Geometry: final body of the model. Coordinates: model frame, mm. Round coordinates to 2 decimals unless told otherwise and drop trailing zeros. Write each loop counter-clockwise with the first axis right and the second up, starting at its lowest first coordinate (ties: lowest second). Pieces come first, ordered by that corner, then holes. Notation, with made-up numbers: (-37, -7) - (-6, -7) arc R12 cw to (-6, 2) - close; hole circle Ø8 at (8, 19.25). An arc over 180 degrees is marked (long way). Use a Markdown table: item, result. Add a question column.
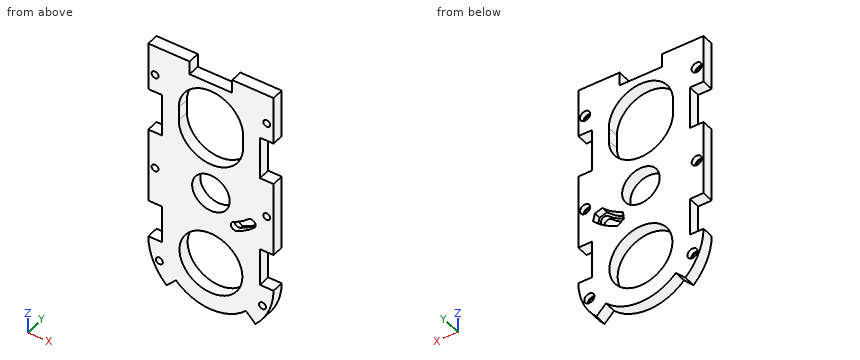
Autodesk Inventor part; units mm, degrees
ref_plane "YZ Plane" through (0, 0, 0) normal (1, 0, 0) x (0, 1, 0)
ref_plane "XZ Plane" through (0, 0, 0) normal (0, 1, 0) x (-1, 0, 0)
ref_plane "XY Plane" through (0, 0, 0) normal (0, 0, 1) x (1, 0, 0)
sketch "Boceto1" plane through (0, 0, 0) normal (0, 1, 0) x (-1, 0, 0)
  line L0 (0, 0) -> (-24.6, 0)
  line L1 (0, 0) -> (0, -29)
  line L2 (0, -29) -> (-8, -29)
  line L3 (-8, -29) -> (-8, -54)
  line L4 (-8, -54) -> (0, -54)
  line L5 (0, -54) -> (0, -99)
  line L6 (0, -99) -> (-8, -99)
  line L7 (-8, -99) -> (-8, -121)
  line L8 (-8, -121) -> (0, -121)
  line L9 (-24.6, 0) -> (-24.6, -8)
  line L10 (-24.6, -8) -> (-49.4, -8)
  line L11 (-37, 21.7087) -> (-37, -150)
  arc A0 (-57.5061, -141.5061) -> (-16.4939, -141.5061) centre (-37, -121) ccw
  line L12 (-37, -121) -> (-16.4939, -141.5061)
  line L13 (-16.4939, -141.5061) -> (-10.837, -147.163)
  line L14 (-74, 0) -> (-49.4, 0)
  line L15 (-74, 0) -> (-74, -29)
  line L16 (-74, -29) -> (-66, -29)
  line L17 (-66, -29) -> (-66, -54)
  line L18 (-66, -54) -> (-74, -54)
  line L19 (-74, -54) -> (-74, -99)
  line L20 (-74, -99) -> (-66, -99)
  line L21 (-66, -99) -> (-66, -121)
  line L22 (-66, -121) -> (-74, -121)
  line L23 (-49.4, 0) -> (-49.4, -8)
  line L24 (-37, -121) -> (-57.5061, -141.5061)
  line L25 (-57.5061, -141.5061) -> (-63.163, -147.163)
  arc A1 (-74, -121) -> (-63.163, -147.163) centre (-37, -121) ccw
  arc A2 (-10.837, -147.163) -> (0, -121) centre (-37, -121) ccw
  dimension "d139" = 24.6
  dimension "d140" = 29
  dimension "d141" = 25
  dimension "d142" = 8
  dimension "d143" = 45
  dimension "d144" = 22
  dimension "d145" = 8
  dimension "d146" = 24.8
  dimension "d148" = 45
extrude "Extrusión1" add sketch "Boceto1" along normal blind 7
sketch "Boceto2" plane through (0, 7, 0) normal (0, 1, 0) x (1, 0, 0)
  arc A0 (18, 32) -> (56, 32) centre (37, 32) ccw
  arc A1 (56, 40) -> (18, 40) centre (37, 40) ccw
  line L0 (18, 40) -> (18, 32)
  line L1 (56, 32) -> (56, 40)
  circle A2 centre (37, 77) radius 11.1
  circle A3 centre (37, 121) radius 18.6
  line L2 (37, -3.2334) -> (37, 158.5758)
  point P0 (0, 0)
  dimension "d18" = 19
  dimension "d23" = 22.2
  dimension "d25" = 37.2
  dimension "d149" = 44
  dimension "d150" = 37
  dimension "d151" = 8
extrude "Extrusión2" cut sketch "Boceto2" against normal blind 7
sketch "Boceto3" plane through (0, 7, 0) normal (0, 1, 0) x (1, 0, 0)
  line L0 (37, -12.6618) -> (37, 178.5268)
  circle A0 centre (4, 18) radius 2.05
  circle A1 centre (4, 76.5) radius 2.05
  circle A2 centre (37, 121) radius 18.6
  circle A3 centre (37, 121) radius 33
  circle A4 centre (6.512, 133.6286) radius 2.05
  line L1 (8, 29) -> (0, 29)
  line L2 (0, 29) -> (0, 0)
  line L3 (0, 99) -> (0, 54)
  line L4 (8, 99) -> (0, 99)
  line L5 (6.512, 133.6286) -> (37, 121)
  line L6 (24.8695, 121) -> (50.3921, 121)
  circle A5 centre (70, 18) radius 2.05
  circle A6 centre (70, 76.5) radius 2.05
  circle A7 centre (67.488, 133.6286) radius 2.05
  line L7 (67.488, 133.6286) -> (37, 121)
  dimension "d157" = 66
  dimension "d152" = 11
  dimension "d153" = 4
  dimension "d154" = 4.1
  dimension "d155" = 4
  dimension "d156" = 22.5
  dimension "d158" = 22.5
extrude "Extrusión3" cut sketch "Boceto3" against normal through all contours A4 A3 | A3 L5 A4 | A3 A4 L5 | A7 L7 A3 | A3 A7 | L7 A7 A3 | A0 | A1 | A5 | A6
sketch "Boceto12" plane through (0, 7, 0) normal (0, 1, 0) x (1, 0, 0)
  circle A0 centre (37, 77) radius 11.1
  circle A1 centre (37, 121) radius 18.6
  arc A2 (60.7956, 85.0881) -> (51.3765, 91.3074) centre (38.4503, 61.4886) ccw
  line L0 (38.4503, 61.4886) -> (60.7956, 85.0881)
  line L1 (38.4503, 61.4886) -> (51.3765, 91.3074)
  line L2 (51.3765, 91.3074) -> (52.4106, 93.693)
  line L3 (60.7956, 85.0881) -> (62.5832, 86.9761)
  line L4 (38.4503, 61.4886) -> (51.3765, 91.3074)
  line L5 (50.3411, 88.9225) -> (50.3424, 88.9219)
  line L6 (59.009, 83.1992) -> (59.008, 83.2002)
  circle A3 centre (51.3765, 91.3074) radius 2.6
  circle A4 centre (60.7956, 85.0881) radius 2.6
  circle A5 centre (38.4503, 61.4886) radius 29.9
  circle A6 centre (38.4503, 61.4886) radius 35.1
  point P0 (0, 0)
  point P1 (59.009, 83.1992)
  dimension "d101" = 0
  dimension "d102" = 20
  dimension "d91" = 65
  dimension "d173" = 5.2
  dimension "d174" = 5.2
extrude "Extrusión10" cut sketch "Boceto12" against normal through all contours A3 L2 L1 | L1 A2 A3 | A3 A2 A4 A5 | L2 A3 A2 | A6 A4 A2 A3 | A4 A2 L0 | L0 L3 A4 | L3 A2 A4
sketch "Boceto13" plane through (0, 7, 0) normal (0, 1, 0) x (1, 0, 0)
  line L0 (47.0857, 93.1674) -> (50.8419, 95.9533)
  line L1 (50.8419, 95.9533) -> (52.9888, 95.0227)
  line L2 (49.7657, 87.5915) -> (47.6203, 88.5215)
  line L3 (47.6203, 88.5215) -> (47.0857, 93.1674)
  line L4 (59.7114, 80.539) -> (57.9998, 82.1579)
  line L5 (63.5861, 88.0233) -> (65.2773, 86.4238)
  line L6 (65.2773, 86.4238) -> (64.1931, 81.8747)
  line L7 (64.1931, 81.8747) -> (59.7114, 80.539)
  circle A0 centre (38.4503, 61.4886) radius 28.45
  circle A1 centre (38.4503, 61.4886) radius 36.55
  point P0 (0, 0)
  point P1 (51.3765, 91.3074)
  point P2 (60.7956, 85.0881)
  point P3 (60.7956, 85.0881)
  point P4 (51.3765, 91.3074)
  point P5 (51.3765, 91.3074)
  point P6 (51.3765, 91.3074)
  point P7 (60.7956, 85.0881)
  point P8 (65.2562, 86.3351)
  point P9 (50.7698, 95.8998)
  dimension "d172" = 8.1
extrude "Extrusión11" cut sketch "Boceto13" against normal blind 4 contours L0 A1 L6 L7 L4 A0 L2 L3 picked at (62.116, 83.8351)
sketch "Boceto15" plane through (0, 7, 0) normal (0, 1, 0) x (1, 0, 0)
  circle A0 centre (4.0687, 18) radius 3
  circle A1 centre (4, 76.5) radius 2.05
  circle A2 centre (4, 76.5) radius 3
  circle A3 centre (6.512, 133.6286) radius 2.05
  circle A4 centre (6.512, 133.6286) radius 3
  circle A5 centre (67.488, 133.6286) radius 2.05
  circle A6 centre (67.488, 133.6286) radius 3
  circle A7 centre (70, 76.5) radius 2.05
  circle A8 centre (70, 76.5) radius 3
  circle A9 centre (70, 18) radius 2.05
  circle A10 centre (70, 18) radius 3
  point P0 (0, 0)
  dimension "d159" = 6
  dimension "d160" = 6
  dimension "d161" = 6
  dimension "d162" = 6
  dimension "d163" = 6
  dimension "d164" = 6
extrude "Extrusión12" cut sketch "Boceto15" against normal blind 3 contours A0 | A1 | A2 | A3 | A4 | A5 | A6 | A7 | A8 | A9 | A10
sketch "Boceto16" plane through (0, 7, 0) normal (0, 1, 0) x (1, 0, 0)
  line L0 (0, 29) -> (0, 0)
  line L1 (0, 29) -> (8, 29)
  line L2 (8, 29) -> (8, 28.8)
  line L3 (8, 28.8) -> (0, 28.8)
  line L4 (0, 28.8) -> (0, 29)
  line L5 (0, 54) -> (8, 54)
  line L6 (0, 54) -> (8, 54)
  line L7 (8, 54) -> (8, 54.2)
  line L8 (8, 54.2) -> (0, 54.2)
  line L9 (0, 54.2) -> (0, 54)
  line L10 (8, 99) -> (0, 99)
  line L11 (0, 99) -> (8, 99)
  line L12 (8, 99) -> (8, 98.8)
  line L13 (8, 98.8) -> (0, 98.8)
  line L14 (0, 98.8) -> (0, 99)
  line L15 (8, 121) -> (8, 99)
  line L16 (8, 121) -> (0, 121)
  line L17 (0, 121) -> (0, 121.2)
  line L18 (0, 121.2) -> (8, 121.2)
  line L19 (8, 121.2) -> (8, 121)
  line L20 (16.4939, 141.5061) -> (10.837, 147.163)
  line L21 (16.4939, 141.5061) -> (16.3525, 141.3647)
  line L22 (16.3525, 141.3647) -> (10.6956, 147.0215)
  line L23 (10.6956, 147.0215) -> (10.837, 147.163)
  line L24 (24.6, 0) -> (24.6, 8)
  line L25 (0, 0) -> (24.6, 0)
  line L26 (24.6, 0) -> (24.6, 0.2)
  line L27 (24.6, 0.2) -> (0, 0.2)
  line L28 (0, 0.2) -> (0, 0)
  line L29 (24.6, 8) -> (49.4, 8)
  line L30 (24.6, 8) -> (24.4, 8)
  line L31 (24.4, 8) -> (24.4, 0)
  line L32 (24.4, 0) -> (24.6, 0)
  line L33 (24.6, 0) -> (24.6, 8)
  line L34 (37, -18.4316) -> (37, 165.7514)
  line L35 (74, 29) -> (74, 0)
  line L36 (74, 29) -> (66, 29)
  line L37 (66, 29) -> (66, 28.8)
  line L38 (66, 28.8) -> (74, 28.8)
  line L39 (74, 28.8) -> (74, 29)
  line L40 (74, 54) -> (66, 54)
  line L41 (74, 54) -> (66, 54)
  line L42 (66, 54) -> (66, 54.2)
  line L43 (66, 54.2) -> (74, 54.2)
  line L44 (74, 54.2) -> (74, 54)
  line L45 (66, 99) -> (74, 99)
  line L46 (74, 99) -> (66, 99)
  line L47 (66, 99) -> (66, 98.8)
  line L48 (66, 98.8) -> (74, 98.8)
  line L49 (74, 98.8) -> (74, 99)
  line L50 (66, 121) -> (66, 99)
  line L51 (66, 121) -> (74, 121)
  line L52 (74, 121) -> (74, 121.2)
  line L53 (74, 121.2) -> (66, 121.2)
  line L54 (66, 121.2) -> (66, 121)
  line L55 (57.5061, 141.5061) -> (63.163, 147.163)
  line L56 (57.5061, 141.5061) -> (57.6475, 141.3647)
  line L57 (57.6475, 141.3647) -> (63.3044, 147.0215)
  line L58 (63.3044, 147.0215) -> (63.163, 147.163)
  line L59 (49.4, 0) -> (49.4, 8)
  line L60 (74, 0) -> (49.4, 0)
  line L61 (49.4, 0) -> (49.4, 0.2)
  line L62 (49.4, 0.2) -> (74, 0.2)
  line L63 (74, 0.2) -> (74, 0)
  line L64 (49.4, 8) -> (49.6, 8)
  line L65 (49.6, 8) -> (49.6, 0)
  line L66 (49.6, 0) -> (49.4, 0)
  line L67 (49.4, 0) -> (49.4, 8)
  line L68 (24.4, 8) -> (49.6, 8)
  line L69 (49.6, 8) -> (49.6, 8.2)
  line L70 (49.6, 8.2) -> (24.4, 8.2)
  line L71 (24.4, 8.2) -> (24.4, 8)
  point P0 (24.4, 0.2)
  point P1 (0, 0.2)
  point P2 (49.6, 0.2)
  dimension "d166" = 8
  dimension "d167" = 0.2
  dimension "d168" = 0.2
  dimension "d169" = 0.2
extrude "Extrusión13" cut sketch "Boceto16" against normal through all
properties part number "Primer segmento - inferior v1.2" material "Plastico PETG"
1) Section B-B, the plane z = -57.5. Return the cut outline in (x, y), then the cut area to 3 significant figures.
2) Material intervals for L1, parallel to Z at x = 37, y = 4.5; L2, parallel to X at y = 0.8, z = -76.5; L3, parallel to Z at x = 33.5, y = 6, sorted ascending. Write a range as from..to.
3) Pin query (flat end, axial travel): P1, Ø5.5, axis at x = 70, z = -18, coming from the +Y side; P2, Ø12, axis at x = 42, z = -27, coming from the -Y side; P3, Ø2, axis at x = 4, y = 3.5, coming from the -Z side. Return the tip coordinate at first contact, or that it passes through.
4) Section A-A, the plane x = 37. Return the cut outline in (y, z), then the cut area to 3 significant figures.
5) Section C-C, the plane z = -18. Return the cut outline in (x, y), then the cut area to 3 significant figures.
Output values:
| question | item | result |
|---|---|---|
| 1 | outline | (0, 0) - (29.6, 0) - (29.6, 7) - (0, 7) - close; (44.4, 0) - (74, 0) - (74, 7) - (44.4, 7) - close |
| 1 | area | 414 mm^2 |
| 2 | L1 | z = -150..-139.6, -102.4..-88.1, -65.9..-59, -13..-8.2 |
| 2 | L2 | x = 0..1.95, 6.05..25.91, 48.09..67.95, 72.05..74 |
| 2 | L3 | z = -149.79..-139.27, -102.73..-87.53, -66.47..-58.67, -13.33..-8.2 |
| 3 | P1 | stops at y = 4 |
| 3 | P2 | passes through |
| 3 | P3 | stops at z = -139.57 |
| 4 | outline | (0, -150) - (7, -150) - (7, -139.6) - (0, -139.6) - close; (0, -102.4) - (7, -102.4) - (7, -88.1) - (0, -88.1) - close; (0, -65.9) - (7, -65.9) - (7, -59) - (0, -59) - close; (0, -13) - (7, -13) - (7, -8.2) - (0, -8.2) - close |
| 4 | area | 255 mm^2 |
| 5 | outline | (0, 0) - (1.95, 0) - (1.95, 4) - (1.07, 4) - (1.07, 7) - (0, 7) - close; (6.05, 0) - (24.15, 0) - (24.15, 7) - (7.07, 7) - (7.07, 4) - (6.05, 4) - close; (49.85, 0) - (67.95, 0) - (67.95, 4) - (67, 4) - (67, 7) - (49.85, 7) - close; (72.05, 0) - (74, 0) - (74, 7) - (73, 7) - (73, 4) - (72.05, 4) - close |
| 5 | area | 269 mm^2 |
